Autodesk Inventor part; units mm, degrees
ref_plane "YZ Plane" through (0, 0, 0) normal (1, 0, 0) x (0, 1, 0)
ref_plane "XZ Plane" through (0, 0, 0) normal (0, 1, 0) x (-1, 0, 0)
ref_plane "XY Plane" through (0, 0, 0) normal (0, 0, 1) x (1, 0, 0)
sketch "Sketch1" plane through (0, 0, 0) normal (0, 0, 1) x (1, 0, 0)
  line L0 (-12.5, -20) -> (12.5, -20)
  line L1 (12.5, -20) -> (12.5, 20)
  line L2 (12.5, 20) -> (-12.5, 20)
  line L3 (-12.5, 20) -> (-12.5, -20)
  line L4 (-12.5, -20) -> (12.5, 20) construction
  line L5 (12.5, -20) -> (-12.5, 20) construction
  line L6 (-11, 18.5) -> (12.5, 18.5)
  line L7 (12.5, -18.5) -> (-11, -18.5)
  line L8 (-11, -18.5) -> (-11, 18.5)
  line L9 (0, 0) -> (-11, 0) construction
  dimension "d0" = 25
  dimension "d1" = 40
  dimension "d18" = 1.5
  dimension "d19" = 1.5
extrude "Extrusion1" add sketch "Sketch1" along normal mid plane 550 contours L3 L2 L1 L6 L8 L7 L0
sketch "Sketch2" plane through (0, 0, 0) normal (1, 0, 0) x (0, 1, 0)
  line L0 (-20, -275) -> (-20, 275)
  line L1 (20, 275) -> (-20, 275)
  line L2 (20, -275) -> (20, 275)
  line L3 (-20, -275) -> (20, -275)
  line L4 (20, -275) -> (3.094, -275) construction
  line L5 (3.094, -275) -> (-20, -235) construction
  spline S0 degree 2 poles (20, -275) (3.094, -275) (-20, -235) knots 1 1 1 2 2 2
  point P0 (0, 0)
  dimension "d7" = 40
  dimension "d8" = 30
extrude "Extrusion2" cut sketch "Sketch2" along normal through all both and the other way through all contours L0 S0 L3
mirror "Mirror1" about plane through (0, 0, 0) normal (0, 0, 1) of "Extrusion2"
sketch "Sketch3" plane through (-12.5, 20, -275) normal (-1, 0, 0) x (0, 0, 1)
  circle A0 centre (275, -20) radius 7
  line L0 (270, -24.899) -> (270, -15.101)
  line L1 (280, -15.101) -> (280, -24.899)
  circle A1 centre (275, -20) radius 12.5
  dimension "d11" = 14
  dimension "d12" = 10
  dimension "d26" = 25
extrude "Extrusion3" cut sketch "Sketch3" against normal up to next contours A0 L1 | L1 A0 L0 | L0 A0
properties part number "profile" material "Aluminum 6061"
For this review, take the finished solid that the model builds, in its own axes (mm). A direction names the side the tool comes from. Round coordinates to 2 decimals unless told otherwise and drop trailing zeros. Loops run counter-clockwise (first coordinate to the right, second up) from the corner with the lowest first, then second, coordinate; pieces in that order, holes last. Notation, with made-up numbers: (27.25, -30.5) - (39.25, -30.5) arc R7 ccw to (39.25, -17.5) - close; hole circle Ø3 at (-22.75, 29.5). An arc over 180 degrees is marked (long way). Put each result on its own line as item: value. Start each with the question number.
1. For faces 3 (the flat face through (-11, 8, -4)), 4 (the flat face through (-12.5, 9, -4)), list the 3-axis set-ups (+Z, -Z, +X, -X, +Y, -Y) from which the entire face can be reached by the end or side of a thin tool; tool diameter is ignored.
2. For probe 1 along Y at (x, z) = (11.25, -41); probe 2 along Y at (x, z) = (-11.6, 0); probe 3 along X at (y, z) = (16, -121.5), list the stretches that pass through material, from the lowest coordinate up. Write a range as [from, to].
3. Consider section B-B on z = -81. State the section outline as (x, y) points.
4. Consider section A-A on z = 0. State the section outline as (x, y) points, plus the area to 4 significant figures.
5. Insertion check: P1, Ø10, axis at y = 5, z = 135, coming from the +X side; P2, Ø8, axis at x = -9, y = -11.5, coming from the +Z side. Each pin has a flat end and moves straight along its axis. Give the tip position at first contact, or say it passes through.
6. Mouldability with a two-part tool opening along Z and no side actions: class faces 1 (the cylindrical face through (-11.76, -2.681, 6.466)), 2 (the flat face through (0, 20, -4)) as +Z half, -Z half, draft (parallel to the pull), parting line (faces both ways), or undercut.
Result sheet:
1. face 3: +Z, -Z, +X
1. face 4: +Z, -Z, -X, +Y, -Y
2. probe 1: [-20, -18.5], [18.5, 20]
2. probe 2: [-20, -7], [7, 20]
2. probe 3: [-12.5, -11]
3. outline: (-12.5, -20) - (12.5, -20) - (12.5, -18.5) - (-11, -18.5) - (-11, 18.5) - (12.5, 18.5) - (12.5, 20) - (-12.5, 20) - close
4. outline: (-12.5, -20) - (12.5, -20) - (12.5, -18.5) - (-11, -18.5) - (-11, -7) - (-12.5, -7) - close; (-12.5, 7) - (-11, 7) - (-11, 18.5) - (12.5, 18.5) - (12.5, 20) - (-12.5, 20) - close
4. area: 109.5 mm^2
5. P1: x = -11
5. P2: z = 253.61
6. face 1: undercut
6. face 2: draft
